Model file for the job. Use its own axes, mm. A direction names the side the tool comes from. Give positions to 0.01 mm unless a question says otherwise; leave off trailing zeros. Loops run counter-clockwise (first coordinate to the right, second up) from the corner with the lowest first, then second, coordinate; pieces in that order, holes last. Notation, with made-up numbers: (3.25, -7.75) - (38.25, -7.75) arc R35 cw to (38.25, 29.25) - close; hole circle Ø3 at (71, 2). An arc over 180 degrees is marked (long way). Answer as CSV lines item,"result". Start each with the question number.
Item 1: Pull direction Z, two halves, no side cores. Call faces 6 (the flat face through (0, 145, -10)), 7 (the flat face through (15, 118, 2)), 8 (the flat face through (-0.21, 236.302, 101.788)): pulls with the +Z half, pulls with the -Z half, needs draft (parallel to the pull), parting line crosses it, or undercut.
Item 2: Drill centre lines: L1, parallel to X at y = 234.5, z = 107; L2, parallel to X at y = 248, z = -4.5; L3, parallel to Z at x = -3, y = 16. Where is each one in solid material? Low to high. Write a range as from..to.
Item 3: Saw through at C-C on x = -150. Give the cut face in (y, z), plus the area to 3 significant figures.
Item 4: Saw through at D-D on y = 177. Give the cut face in (x, z), plus the area to 3 significant figures.
Item 5: Saw through at B-B on y = 0. Give the cut face in (x, z).
Item 6: Pin check, flat tips, straight feed: pin 1 (24 mm diameter, centred on x = 0, y = 151, fed in from +Z); pin 2 (21.5 mm diameter, centred on y = 225.5, z = 120.5, fed in from -X); pin 3 (13 mm diameter, centred on y = 224, z = 136.5, fed in from +X). Stop position of each tip, or through.
Item 7: Tool access for faces 1 (the cylindrical face through (-0.21, 261.013, 45.798)), 2 (the cylindrical face through (-98.655, 0.33, 7.493)), 3 (the cylindrical face through (96.345, 0.33, 7.493)), 4 (the flat face through (-15, 238, 137)), 5 (the flat face through (-0.28, 253.712, 145.915)): list every direction of +Z, -Z, +X, -X, +Y, -Y with a clear straight run to the whole face (end or side of a thin tool).
Item 8: Saw through at A-A on z = 0. Give the cut face in (x, y), plus the area to 3 significant figures.
from build123d import *
from build123d.topology import SkipClean

# Parameters (mm, degrees)
BOSS_EXTRUDE1_DEPTH             = 15
BOSS_EXTRUDE1_DEPTH_BACK        = 15
BOSS_EXTRUDE3_REACH             = 306.228
BOSS_EXTRUDE3_END_RADIUS        = 250
SKETCH5_W                       = 40
SKETCH5_H                       = 70
BOSS_EXTRUDE3_DIRECTION_2_DEPTH = 30
SKETCH6_W                       = 30
SKETCH6_H                       = 25
CUT_EXTRUDE2_DEPTH              = 70
CUT_EXTRUDE3_REACH              = 306.515
CUT_EXTRUDE3_END_RADIUS         = 250
SKETCH7_W                       = 30.021890818
SKETCH7_H                       = 60
CUT_EXTRUDE4_REACH              = 327.352
SKETCH8_R                       = 2.5
CUT_EXTRUDE4_DIRECTION_2_REACH  = 327.352
BOSS_EXTRUDE4_DEPTH             = 180
BOSS_EXTRUDE4_DEPTH_BACK        = 180
SKETCH11_R                      = 7.5


with BuildPart() as part:
    # Sketch1 → Boss-Extrude1 (new, two sides: drawn at the far end of the back side and taken through both)
    with BuildSketch(Plane(origin=(0, 0, 0), x_dir=(0, 0, -1), z_dir=(1, 0, 0)).offset(-BOSS_EXTRUDE1_DEPTH_BACK)):
        with BuildLine():
            Line((10, 28.284271247), (10, 264.811253537))
            ThreePointArc((10, 264.811253537), (-46.581095136, 260.873918926), (-101.028366233, 244.986263322))
            Line((-101.028366233, 244.986263322), (-161.650144498, 209.986263322))
            Line((-161.650144498, 209.986263322), (-152.500136319, 198.100248417))
            ThreePointArc((-152.500136319, 198.100248417), (-85.263049352, 235.011089984), (-10, 249.799919936))
            Line((-10, 249.799919936), (-10, 28.284271247))
            ThreePointArc((-10, 28.284271247), (0, -30), (10, 28.284271247))
        make_face()
    extrude(amount=BOSS_EXTRUDE1_DEPTH + BOSS_EXTRUDE1_DEPTH_BACK)

    # Boss-Extrude3: up to this cylinder (the profile starts outside it)
    with SkipClean():  # the faces are left unmerged after this step: merging them gives an invalid solid
        boss_extrude3_end = Plane(origin=(0, 0, 0), z_dir=(-1, 0, 0)) * Cylinder(BOSS_EXTRUDE3_END_RADIUS, 1113.456, mode=Mode.PRIVATE)
        # Sketch5 → Boss-Extrude3 (add, up to the surface)
        with BuildSketch(Plane(origin=(0, 227.486263322, 131.339255366), x_dir=(1, 0, 0), z_dir=(0, 0.8660254037844353, 0.5000000000000059)), mode=Mode.PRIVATE) as boss_extrude3_sk1:
            Rectangle(SKETCH5_W, SKETCH5_H)
        boss_extrude3_tool1 = extrude(boss_extrude3_sk1.sketch, amount=-BOSS_EXTRUDE3_REACH, mode=Mode.PRIVATE) - boss_extrude3_end
        add(boss_extrude3_tool1.solids().sort_by_distance((0, 227.486263, 131.339255))[0])

    # Sketch5 → Boss-Extrude3 direction 2 (add)
    with SkipClean():  # the faces are left unmerged after this step: merging them gives an invalid solid
        with BuildSketch(Plane(origin=(0, 227.486263322, 131.339255366), x_dir=(1, 0, 0), z_dir=(0, 0.8660254037844353, 0.5000000000000059))):
            Rectangle(SKETCH5_W, SKETCH5_H)
        extrude(amount=BOSS_EXTRUDE3_DIRECTION_2_DEPTH)

    # Sketch6 → Cut-Extrude2 (cut)
    with SkipClean():  # the faces are left unmerged after this step: merging them gives an invalid solid
        with BuildSketch(Plane(origin=(0, 17.5, -30.310889132), x_dir=(-1, 0, 0), z_dir=(0, 0.5000000000000059, -0.8660254037844353))):
            with Locations((0, 275.178510731)):
                Rectangle(SKETCH6_W, SKETCH6_H)
        extrude(amount=-CUT_EXTRUDE2_DEPTH, mode=Mode.SUBTRACT)

    # Cut-Extrude3: up to this cylinder (the profile starts outside it)
    cut_extrude3_end = Plane(origin=(0, 0, 0), z_dir=(-1, 0, 0)) * Cylinder(CUT_EXTRUDE3_END_RADIUS, 1114.03, mode=Mode.PRIVATE)
    # Sketch7 → Cut-Extrude3 (cut, up to the surface)
    with BuildSketch(Plane(origin=(0, 227.486263322, 131.339255366), x_dir=(1, 0, 0), z_dir=(0, 0.8660254037844353, 0.5000000000000059)), mode=Mode.PRIVATE) as cut_extrude3_sk1:
        Rectangle(SKETCH7_W, SKETCH7_H)
    cut_extrude3_tool1 = extrude(cut_extrude3_sk1.sketch, amount=-CUT_EXTRUDE3_REACH, mode=Mode.PRIVATE) - cut_extrude3_end
    add(cut_extrude3_tool1.solids().sort_by_distance((0, 227.486263, 131.339255))[0], mode=Mode.SUBTRACT)

    # Cut-Extrude4: up to this face of the body (flat: up to its plane)
    cut_extrude4_end = Plane(part.part.faces().sort_by_distance((-20, 234.626657577, 135.461763911))[0])
    # Sketch8 → Cut-Extrude4 (cut, up to the picked face)
    with BuildSketch(Plane(origin=(-15.010945409, 0, 0), x_dir=(0, 0, -1), z_dir=(1, 0, 0)), mode=Mode.PRIVATE) as cut_extrude4_sk1:
        with Locations((-128.169627683, 221.996307134)):
            Circle(SKETCH8_R)
    cut_extrude4_tool1 = split(extrude(cut_extrude4_sk1.sketch, amount=-CUT_EXTRUDE4_REACH, mode=Mode.PRIVATE), bisect_by=cut_extrude4_end, keep=Keep.BOTH, mode=Mode.PRIVATE)
    add(cut_extrude4_tool1.solids().sort_by(Axis((-15.010945, 221.996307, 128.169628), (-1, 0, 0)))[0], mode=Mode.SUBTRACT)

    # Cut-Extrude4 direction 2: up to this face of the body (flat: up to its plane)
    cut_extrude4_direction_2_end = Plane(part.part.faces().sort_by_distance((20, 234.626657577, 135.461763911))[0])
    # Sketch8 → Cut-Extrude4 direction 2 (cut, up to the picked face)
    with BuildSketch(Plane(origin=(-15.010945409, 0, 0), x_dir=(0, 0, -1), z_dir=(1, 0, 0)), mode=Mode.PRIVATE) as cut_extrude4_direction_2_sk1:
        with Locations((-128.169627683, 221.996307134)):
            Circle(SKETCH8_R)
    cut_extrude4_direction_2_tool1 = split(extrude(cut_extrude4_direction_2_sk1.sketch, amount=CUT_EXTRUDE4_DIRECTION_2_REACH, mode=Mode.PRIVATE), bisect_by=cut_extrude4_direction_2_end, keep=Keep.BOTH, mode=Mode.PRIVATE)
    add(cut_extrude4_direction_2_tool1.solids().sort_by(Axis((-15.010945, 221.996307, 128.169628), (1, 0, 0)))[0], mode=Mode.SUBTRACT)

    # Sketch11 → Boss-Extrude4 (add, two sides: drawn at the far end of the back side and taken through both)
    with BuildSketch(Plane(origin=(0, 0, 0), x_dir=(0, 0, -1), z_dir=(1, 0, 0)).offset(-BOSS_EXTRUDE4_DEPTH_BACK)):
        Circle(SKETCH11_R)
    extrude(amount=BOSS_EXTRUDE4_DEPTH + BOSS_EXTRUDE4_DEPTH_BACK)


solid = part.part
Responses:
1,face 6,"pulls with the -Z half"
1,face 7,"needs draft"
1,face 8,"undercut"
2,L1,"-20..-15.01, 15.01..20"
2,L2,"-15..15"
2,L3,"-25.38..25.38"
3,outline,"circle Ø15 at (0, 0)"
3,area,"177 mm2"
4,outline,"(-15, -10) - (15, -10) - (15, 10) - (-15, 10) - close"
4,area,"600 mm2"
5,outline,"(-180, -7.5) - (-15, -7.5) - (-15, -30) - (15, -30) - (15, -7.5) - (180, -7.5) - (180, 7.5) - (15, 7.5) - (15, 30) - (-15, 30) - (-15, 7.5) - (-180, 7.5) - close"
6,pin 1,"z = 10"
6,pin 2,"x = -20"
6,pin 3,"x = 20"
7,face 1,"+X, -X, +Y"
7,face 2,"-X"
7,face 3,"+X"
7,face 4,"none"
7,face 5,"+Z, +X, -X, +Y"
8,outline,"(-180, -7.5) - (-15, -7.5) - (-15, -30) - (15, -30) - (15, -7.5) - (180, -7.5) - (180, 7.5) - (15, 7.5) - (15, 265) - (-15, 265) - (-15, 7.5) - (-180, 7.5) - close"
8,area,"13,800 mm2"
